Verification items for the finished model (mm, model axes). A direction names the side the tool comes from. Coordinates: 2 decimals unless noted, no trailing zeros. Order: outer loops, then holes, each group sorted by start corner. A loop starts at its lowest first (then second) coordinate and runs counter-clockwise, first axis right, second up. Notation, with made-up numbers: M 51.5,51.5 L 78.5,51.5 A20 cw 78.5,74.5 Z; hole C 15.25,-32 d6. An arc over 180 degrees is marked long. Return JSON: item names as keys, results as strings.
Autodesk Inventor part; units mm, degrees
ref_plane "YZ Plane" through (0, 0, 0) normal (1, 0, 0) x (0, 1, 0)
ref_plane "XZ Plane" through (0, 0, 0) normal (0, 1, 0) x (-1, 0, 0)
ref_plane "XY Plane" through (0, 0, 0) normal (0, 0, 1) x (1, 0, 0)
sketch "スケッチ1" plane through (0, 0, 0) normal (0, 1, 0) x (-1, 0, 0)
  circle A0 centre (0, 0) radius 10
  line L0 (0, 10) -> (-10, 10)
  line L1 (-10, 10) -> (-10, -10)
  line L2 (-10, -10) -> (10, -10)
  line L3 (10, -10) -> (10, 0)
  dimension "d0" = 20
  dimension "d1" = 10
  dimension "d2" = 10
extrude "押し出し1" add sketch "スケッチ1" along normal mid plane 77
sketch "スケッチ2" plane through (0, -38.5, 10) normal (0, 0, 1) x (1, 0, 0)
  line L0 (10, 0) -> (10, 77)
  line L1 (0, 77) -> (10, 77)
  line L2 (0, 0) -> (0, 77)
  line L3 (10, 0) -> (0, 0)
extrude "押し出し2" cut sketch "スケッチ2" against normal blind 1
sketch "スケッチ3" plane through (-10, -38.5, -10) normal (-1, 0, 0) x (0, 0, 1)
  line L0 (0, 77) -> (10, 77)
  line L1 (10, 0) -> (10, 77)
  line L2 (10, 0) -> (0, 0)
  line L3 (0, 0) -> (0, 77)
  point P0 (10, 38.5)
extrude "押し出し3" cut sketch "スケッチ3" against normal blind 1
sketch "スケッチ4" plane through (0, -38.5, 9) normal (0, 0, 1) x (1, 0, 0)
  line L0 (0, 77) -> (10, 77)
  line L1 (10, 77) -> (10, 0)
  line L2 (10, 0) -> (0, 0)
  point P0 (0, 38.5)
  point P1 (5, 72)
  point P2 (5, 5)
  dimension "d9" = 5
  dimension "d10" = 5
  dimension "d11" = 5
hole "穴1" at (5, 33.5, 9) at (5, -33.5, 9) direction (0, 0, -1) diameter 5 depth 6 tip angle 118
sketch "スケッチ5" plane through (0, -38.5, 0) normal (0, 1, 0) x (1, 0, 0)
  point P0 (0, 0)
hole "穴2" at (0, -38.5, 0) direction (0, 1, 0) diameter 5 depth 6 tip angle 118
sketch "スケッチ6" plane through (-9, -38.5, -10) normal (-1, 0, 0) x (0, 0, 1)
  line L0 (0, 0) -> (0, 77)
  line L1 (0, 77) -> (10, 77)
  line L2 (10, 0) -> (0, 0)
  point P0 (10, 38.5)
  point P1 (5, 72)
  point P2 (5, 5)
  dimension "d26" = 5
  dimension "d27" = 5
  dimension "d28" = 5
  dimension "d29" = 5
hole "穴3" at (-9, 33.5, -5) at (-9, -33.5, -5) direction (1, 0, 0) diameter 5 depth 6 tip angle 118
mirror "ミラー1" about plane through (0, 0, 0) normal (0, 1, 0) of "穴2"
sketch "スケッチ9" plane through (10, -38.5, -10) normal (1, 0, 0) x (0, 0, -1)
  line L0 (0, 77) -> (-10, 77)
  line L1 (-19, 77) -> (-19, 0)
  line L2 (0, 77) -> (-19, 77)
  line L3 (-19, 77) -> (-19, 62)
  line L4 (-19, 62) -> (0, 62)
  line L5 (0, 62) -> (0, 77)
  point P0 (-10, 38.5)
  dimension "d47" = 15
extrude "押し出し6" add sketch "スケッチ9" along normal blind 20
sketch "スケッチ10" plane through (0, 38.5, 0) normal (0, 1, 0) x (1, 0, 0)
  line L0 (30, 10) -> (30, -9)
  point P0 (0, 0)
  point P1 (20, 0)
  dimension "d50" = 10
hole "穴4" at (20, 38.5, 0) direction (0, -1, 0) diameter 6.1 depth 6
chamfer "面取り2" distance 3 angle 45 1 edges at (20, 38.5, -3.05)
chamfer "面取り3" distance 20 angle 45 1 edges at (10, 23.5, -0.5)
properties part number "base8" material "ABS プラスチック"
Q1. Draft check along Z on faces 1 (the face through (16.839, 35.688, -0.702)), 2 (the face through (2.52, -33.17, 5.96)), 3 (the face through (6, 8, -10)). Enter one of: pulls with the +Z half, pulls with the -Z half, needs draft (parallel to the pull), parting line crosses it, or undercut.
Values:
{"face 1": "undercut", "face 2": "needs draft", "face 3": "pulls with the -Z half"}
Q2. Cross-section at C-C, the plane x = -4. Record the boundary of the cut face in (y, z).
Values:
{"outline": "M -38.5,-10 L 38.5,-10 L 38.5,9.17 L -38.5,9.17 Z; hole C -33.5,-5 d5; hole C 33.5,-5 d5"}
Q3. Material ranges on line 1 along Y through (x, z) = (-5.25, -5); line 2 along Z through (x, y) = (3, 3); line 3 along X through (y, z) = (33, 4), recorded low to high.
Values:
{"line 1": "-38.5 to -36, -31 to 31, 36 to 38.5", "line 2": "-10 to 9", "line 3": "-9.17 to 2.55, 7.45 to 30"}
Q4. Cross-section at B-B, the plane y = 25.5. Record the boundary of the cut face in (x, z).
Values:
{"outline": "M -10,0 L -9,0 L -9,-10 L 30,-10 L 30,9 L 0,9 L 0,10 A10 ccw Z"}
Q5. Tool access check on faces 4 (the face through (-5.96, 31.39, -3.66)), 5 (the face through (-2.44, 35.46, 0.54)), 6 (the face through (-9, 1, -5)). Record the directions out of +Z, -Z, +X, -X, +Y, -Y that give a thin tool (end or side, any length) a straight path to the whole face; none if there is none.
Values:
{"face 4": "-X", "face 5": "+Y", "face 6": "-Z, -X, +Y, -Y"}
Q6. Cross-section at D-D, the plane x = 20. Record the boundary of the cut face in (y, z), and give its area (3 significant figures).
Values:
{"outline": "M 13.5,-10 L 38.5,-10 L 38.5,-6.05 L 35.5,-3.05 L 32.5,-3.05 L 32.5,3.05 L 35.5,3.05 L 38.5,6.05 L 38.5,9 L 13.5,9 Z", "area": "429 mm^2"}
Q7. Cross-section at A-A, the plane z = 7. State how many separate pieces and enclosed holes the cut face has, and give its area (3 significant figures).
Values:
{"separate pieces": "1", "enclosed holes": "2", "area": "1,780 mm^2"}
Q8. Go/stop test with flat-tipped pins: pin 1 (3 mm diameter, centred on x = 5, y = 33.5, fed in from +Z); pin 2 (2 mm diameter, centred on y = 17.5, z = 3, fed in from -X); pin 3 (6.5 mm diameter, centred on x = 18.5, z = 0, fed in from +Y). Record where each tip stops, or that it passes through.
Values:
{"pin 1": "z = 2.4", "pin 2": "x = -9.8", "pin 3": "y = 37.2"}
